from build123d import *

# Parameters (mm, degrees)
SKETCH_1_W           = 25
SKETCH_1_H           = 30
SKETCH_1_W_2         = 23
SKETCH_1_H_2         = 28
EXTRUDE_1_DEPTH      = 242.5
SKETCH_4_R           = 1.5
CUT_EXTRUDE_3_DEPTH  = 5
SKETCH_5_R           = 1.525
CUT_EXTRUDE_4_DEPTH  = 80
SKETCH_8_R           = 1.55
CUT_EXTRUDE_5_DEPTH  = 59
SKETCH_9_R           = 1.505
CUT_EXTRUDE_6_DEPTH  = 51
CUT_EXTRUDE_7_DEPTH  = 146
SKETCH_11_R          = 2
CUT_EXTRUDE_8_DEPTH  = 39.5
CUT_EXTRUDE_11_REACH = 246.246
SKETCH_13_R          = 2


with BuildPart() as part:
    # 草图1 → 凸台-拉伸1 (new, symmetric)
    with BuildSketch(Plane.XY):
        Rectangle(SKETCH_1_W, SKETCH_1_H)
        Rectangle(SKETCH_1_W_2, SKETCH_1_H_2, mode=Mode.SUBTRACT)
    extrude(amount=EXTRUDE_1_DEPTH, both=True)

    # 草图4 → 切除-拉伸3 (cut, symmetric)
    with BuildSketch(Plane.XZ.offset(-14)):
        with Locations((7.5, 214.55)):
            Circle(SKETCH_4_R)
        with Locations((-7.5, 214.55)):
            Circle(SKETCH_4_R)
        with Locations((7.5, 230.55)):
            Circle(SKETCH_4_R)
        with Locations((-7.5, 230.55)):
            Circle(SKETCH_4_R)
        with Locations((7.5, 124.65)):
            Circle(SKETCH_4_R)
        with Locations((7.5, 140.65)):
            Circle(SKETCH_4_R)
        with Locations((-7.5, 140.65)):
            Circle(SKETCH_4_R)
        with Locations((-7.5, 124.65)):
            Circle(SKETCH_4_R)
    extrude(amount=CUT_EXTRUDE_3_DEPTH, both=True, mode=Mode.SUBTRACT)

    # 草图5 → 切除-拉伸4 (cut, symmetric)
    with BuildSketch(Plane(origin=(0, 15, 0), x_dir=(1, 0, 0), z_dir=(0, 1, 0))):
        with Locations((-7.5, -163.6)):
            Circle(SKETCH_5_R)
        with Locations((7.5, -163.6)):
            Circle(SKETCH_5_R)
        with Locations((-7.5, -191.6)):
            Circle(SKETCH_5_R)
        with Locations((7.5, -191.6)):
            Circle(SKETCH_5_R)
    extrude(amount=CUT_EXTRUDE_4_DEPTH, both=True, mode=Mode.SUBTRACT)

    # 草图8 → 切除-拉伸5 (cut)
    with BuildSketch(Plane(origin=(0, 15, 0), x_dir=(1, 0, 0), z_dir=(0, 1, 0))):
        with Locations(Location((8.5, 236.5, 0), (0, 0, 270))):
            Circle(SKETCH_8_R)
        with Locations(Location((-8.5, 236.5, 0), (0, 0, 270))):
            Circle(SKETCH_8_R)
        with Locations(Location((-8.5, 216.5, 0), (0, 0, 270))):
            Circle(SKETCH_8_R)
        with Locations(Location((8.5, 216.5, 0), (0, 0, 270))):
            Circle(SKETCH_8_R)
    extrude(amount=-CUT_EXTRUDE_5_DEPTH, mode=Mode.SUBTRACT)

    # 草图9 → 切除-拉伸6 (cut)
    with BuildSketch(Plane(origin=(12.5, 0, 0), x_dir=(0, 0, -1), z_dir=(1, 0, 0))):
        with Locations((103.4, -11)):
            Circle(SKETCH_9_R)
        with Locations((103.4, 11)):
            Circle(SKETCH_9_R)
        with Locations((81.4, 11)):
            Circle(SKETCH_9_R)
        with Locations((81.4, -11)):
            Circle(SKETCH_9_R)
        with Locations((-44.295, -11)):
            Circle(SKETCH_9_R)
        with Locations((-44.295, 11)):
            Circle(SKETCH_9_R)
        with Locations((-22.295, 11)):
            Circle(SKETCH_9_R)
        with Locations((-22.295, -11)):
            Circle(SKETCH_9_R)
        with Locations((-107.4, -11)):
            Circle(SKETCH_9_R)
        with Locations((-129.4, -11)):
            Circle(SKETCH_9_R)
        with Locations((-107.4, 11)):
            Circle(SKETCH_9_R)
        with Locations((-129.4, 11)):
            Circle(SKETCH_9_R)
    extrude(amount=-CUT_EXTRUDE_6_DEPTH, mode=Mode.SUBTRACT)

    # 草图10 → 切除-拉伸7 (cut)
    with BuildSketch(Plane.ZY.offset(12.5)):
        with BuildLine():
            Line((-51.4, 6), (-7.705, 6))
            ThreePointArc((-7.705, 6), (-1.705, 0), (-7.705, -6))
            Line((-7.705, -6), (-51.4, -6))
            ThreePointArc((-51.4, -6), (-57.4, 0), (-51.4, 6))
        make_face()
        with BuildLine():
            Line((62.295, 6), (89.4, 6))
            ThreePointArc((89.4, 6), (95.4, 0), (89.4, -6))
            Line((89.4, -6), (62.295, -6))
            ThreePointArc((62.295, -6), (56.295, 0), (62.295, 6))
        make_face()
    extrude(amount=-CUT_EXTRUDE_7_DEPTH, mode=Mode.SUBTRACT)

    # 草图11 → 切除-拉伸8 (cut, symmetric)
    with BuildSketch(Plane(origin=(12.5, 0, 0), x_dir=(0, 0, -1), z_dir=(1, 0, 0))):
        with Locations((156.5, 9.5)):
            Circle(SKETCH_11_R)
        with Locations((126.5, 9.5)):
            Circle(SKETCH_11_R)
        with Locations((126.5, -9.5)):
            Circle(SKETCH_11_R)
        with Locations((156.5, -9.5)):
            Circle(SKETCH_11_R)
    extrude(amount=CUT_EXTRUDE_8_DEPTH, both=True, mode=Mode.SUBTRACT)

    # 切除-拉伸11: up to this face of the body (flat: up to its plane)
    cut_extrude_11_end = Plane(part.part.faces().sort_by_distance((-12.5, 0, -0.673656222))[0])
    # 草图13 → 切除-拉伸11 (cut, up to the picked face)
    with BuildSketch(Plane(origin=(12.5, 0, 0), x_dir=(0, 0, -1), z_dir=(1, 0, 0)), mode=Mode.PRIVATE) as cut_extrude_11_sk1:
        with Locations((-144, -9.5)):
            Circle(SKETCH_13_R)
    cut_extrude_11_tool1 = split(extrude(cut_extrude_11_sk1.sketch, amount=-CUT_EXTRUDE_11_REACH, mode=Mode.PRIVATE), bisect_by=cut_extrude_11_end, keep=Keep.BOTH, mode=Mode.PRIVATE)
    # 草图13 → 切除-拉伸11 (cut, up to the picked face)
    with BuildSketch(Plane(origin=(12.5, 0, 0), x_dir=(0, 0, -1), z_dir=(1, 0, 0)), mode=Mode.PRIVATE) as cut_extrude_11_sk2:
        with Locations((-144, 9.5)):
            Circle(SKETCH_13_R)
    cut_extrude_11_tool2 = split(extrude(cut_extrude_11_sk2.sketch, amount=-CUT_EXTRUDE_11_REACH, mode=Mode.PRIVATE), bisect_by=cut_extrude_11_end, keep=Keep.BOTH, mode=Mode.PRIVATE)
    # 草图13 → 切除-拉伸11 (cut, up to the picked face)
    with BuildSketch(Plane(origin=(12.5, 0, 0), x_dir=(0, 0, -1), z_dir=(1, 0, 0)), mode=Mode.PRIVATE) as cut_extrude_11_sk3:
        with Locations((-174, -9.5)):
            Circle(SKETCH_13_R)
    cut_extrude_11_tool3 = split(extrude(cut_extrude_11_sk3.sketch, amount=-CUT_EXTRUDE_11_REACH, mode=Mode.PRIVATE), bisect_by=cut_extrude_11_end, keep=Keep.BOTH, mode=Mode.PRIVATE)
    # 草图13 → 切除-拉伸11 (cut, up to the picked face)
    with BuildSketch(Plane(origin=(12.5, 0, 0), x_dir=(0, 0, -1), z_dir=(1, 0, 0)), mode=Mode.PRIVATE) as cut_extrude_11_sk4:
        with Locations((-174, 9.5)):
            Circle(SKETCH_13_R)
    cut_extrude_11_tool4 = split(extrude(cut_extrude_11_sk4.sketch, amount=-CUT_EXTRUDE_11_REACH, mode=Mode.PRIVATE), bisect_by=cut_extrude_11_end, keep=Keep.BOTH, mode=Mode.PRIVATE)
    add(cut_extrude_11_tool1.solids().sort_by(Axis((12.5, -9.5, 144), (-1, 0, 0)))[0], mode=Mode.SUBTRACT)
    add(cut_extrude_11_tool2.solids().sort_by(Axis((12.5, 9.5, 144), (-1, 0, 0)))[0], mode=Mode.SUBTRACT)
    add(cut_extrude_11_tool3.solids().sort_by(Axis((12.5, -9.5, 174), (-1, 0, 0)))[0], mode=Mode.SUBTRACT)
    add(cut_extrude_11_tool4.solids().sort_by(Axis((12.5, 9.5, 174), (-1, 0, 0)))[0], mode=Mode.SUBTRACT)


solid = part.part
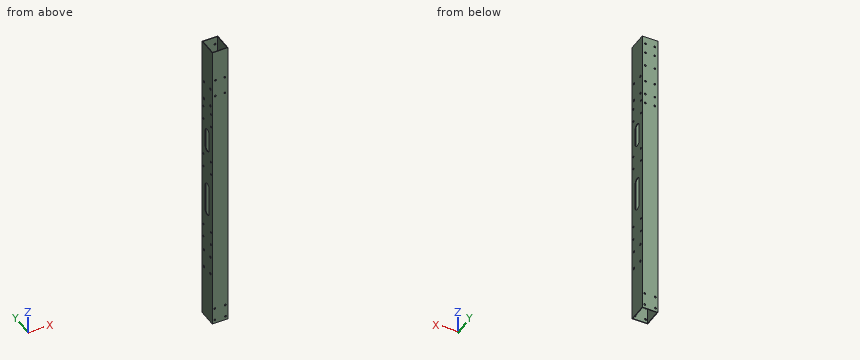
Geometry check sheet. Reference: the model listing, model coordinates, mm. Round coordinates to 2 decimals unless told otherwise and drop trailing zeros. Order: outer loops, then holes, each group sorted by start corner. A loop starts at its lowest first (then second) coordinate and runs counter-clockwise, first axis right, second up. Notation, with made-up numbers: (-21, 4.5) - (-15, 4.5) arc R22 ccw to (-15, 31.5) - close; hole circle Ø3 at (88.5, 7.25). An arc over 180 degrees is marked (long way). One line per question, with ' | ' between items. Start each with the question number.
(1) Sectioned sample at A-A on x = -0.25. Record the cut outline in (y, z), and give its area (3 significant figures).
(2) Thickness scan on L1, parallel to Y at x = -11.85, z = 129.4 (3 decimals); L2, parallel to X at y = 14.7, z = 140.65; L3, parallel to Y at x = -6.5, z = 135. Record the ranges inside material, lowest first. Write a range as [from, to].
(3) Sectioned sample at B-B on z = -191. Record the cut outline in (x, y).
Conclusion:
1) outline: (-15, -242.5) - (-14, -242.5) - (-14, 242.5) - (-15, 242.5) - close; (14, -242.5) - (15, -242.5) - (15, 242.5) - (14, 242.5) - close | area: 970 mm2
2) L1: y = [-15, -12.505], [-9.495, 9.495], [12.505, 15] | L2: x = [-12.5, -9], [-6, 6], [9, 12.5] | L3: y = [-15, -14], [14, 15]
3) outline: (-12.5, -15) - (12.5, -15) - (12.5, 15) - (-12.5, 15) - close; hole (-11.5, -14) - (11.5, -14) - (11.5, 14) - (-11.5, 14) - close
